Model file for the job. Use its own axes, mm. Round coordinates to 2 decimals unless told otherwise and drop trailing zeros. Order: outer loops, then holes, each group sorted by start corner. A loop starts at its lowest first (then second) coordinate and runs counter-clockwise, first axis right, second up. Notation, with made-up numbers: (2.25, 73) - (34.25, 73) arc R11 cw to (34.25, 79) - close; hole circle Ø1 at (58, 30.25). An arc over 180 degrees is marked (long way). Put each result on its own line as item: value. Start each with the question number.
Item 1: Probe probe 1 along X at (y, z) = (6.75, 3.5); probe 2 along Z at (x, y) = (411.5, 0); probe 3 along X at (y, z) = (5.75, 33). List the from-to ranges inside material, lowest first.
Item 2: Saw through at C-C on x = -34.5. List the corners of the cut face in (y, z), plus the area to 3 significant figures.
Item 3: Saw through at B-B on x = 116. List the corners of the cut face in (y, z).
Item 4: Pin check, flat tips, straight feed: pin 1 Ø6 at (x, z) = (-301, 43) entering from -Y; pin 2 Ø0.9 at (x, y) = (-287.5, 6.5) entering from -Z; pin 3 Ø4 at (x, y) = (-153.5, 6) entering from -Z. Stop position of each tip, or through.
Item 5: Saw through at A-A on y = -2. State how many separate pieces and enclosed holes the cut face has, plus the area to 3 significant figures.
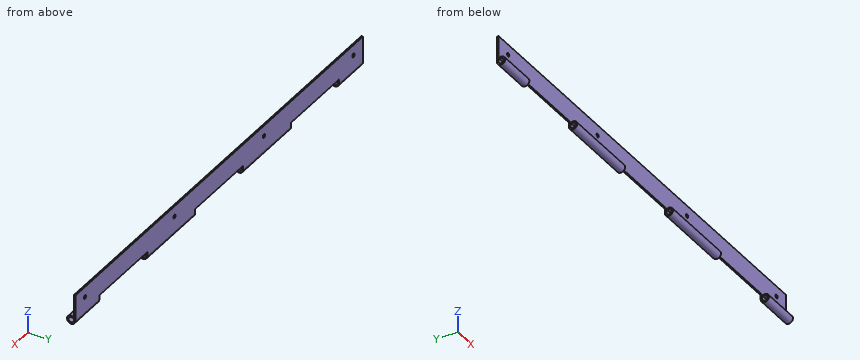
```python
from build123d import *

# Parameters (mm, degrees)
F1_DEPTH  = 450
F9_W      = 16.4
F9_H      = 16.4
F10_DEPTH = 150
F11_W     = 16.4
F11_H     = 16.4
F12_DEPTH = 150
F13_W     = 16.4
F13_H     = 16.4
F14_DEPTH = 150
F15_R     = 3.5
F16_DEPTH = 8.001


with BuildPart() as f1:
    # F0 (on Right) → F1 (new body, symmetric)
    with BuildSketch(Plane.YZ):
        with BuildLine():
            Line((2.867882, 4.09576), (4.588611, 6.553216))
            ThreePointArc((4.588611, 6.553216), (-7.096087, -3.693989), (8, 0))
            Line((8, 0), (8, 50))
            Line((8, 50), (5, 50))
            Line((5, 50), (5, 0))
            ThreePointArc((5, 0), (-4.435054, -2.308743), (2.867882, 4.09576))
        make_face()
    extrude(amount=F1_DEPTH, both=True)

    # F9 (on offset) → F10 (cut)
    with BuildSketch(Plane.YZ.offset(375)):
        Rectangle(F9_W, F9_H)
    extrude(amount=-F10_DEPTH, mode=Mode.SUBTRACT)

    # F11 (on offset) → F12 (cut)
    with BuildSketch(Plane.YZ.offset(75)):
        Rectangle(F11_W, F11_H)
    extrude(amount=-F12_DEPTH, mode=Mode.SUBTRACT)

    # F13 (on offset) → F14 (cut)
    with BuildSketch(Plane.YZ.offset(-225)):
        Rectangle(F13_W, F13_H)
    extrude(amount=-F14_DEPTH, mode=Mode.SUBTRACT)

    # F15 (on Front) → F16 (cut, through all)
    with BuildSketch(Plane.XZ):
        with Locations((140, 30)):
            Circle(F15_R)
        with Locations((-140, 30)):
            Circle(F15_R)
        with Locations((-420, 30)):
            Circle(F15_R)
        with Locations((420, 30)):
            Circle(F15_R)
    extrude(amount=-F16_DEPTH, mode=Mode.SUBTRACT)


solid = f1.part
```
Results found:
1. probe 1: x = -450 to -375, -225 to -75, 75 to 225, 375 to 450
1. probe 2: z = -8 to -5, 5 to 8
1. probe 3: x = -450 to -421.8, -418.2 to -141.8, -138.2 to 138.2, 141.8 to 418.2, 421.8 to 450
2. outline: (5, 8.2) - (8, 8.2) - (8, 50) - (5, 50) - close
2. area: 125 mm²
3. outline: (2.87, 4.1) - (4.59, 6.55) arc R8 ccw (long way) to (8, 0) - (8, 50) - (5, 50) - (5, 0) arc R5 cw (long way) to start
4. pin 1: stops at y = 5
4. pin 2: stops at z = 8.2
4. pin 3: stops at z = -6.93
5. separate pieces: 8
5. enclosed holes: 0
5. area: 2,850 mm²
